CAD build for the part. Positions are in the model's coordinates, mm. Round coordinates to 2 decimals unless told otherwise and drop trailing zeros. Write each loop counter-clockwise with the first axis right and the second up, starting at its lowest first coordinate (ties: lowest second). Pieces come first, ordered by that corner, then holes. Notation, with made-up numbers: (32, 9) - (54, 9) arc R15 cw to (54, 23) - close; hole circle Ø5 at (-7, 4.25). An arc over 180 degrees is marked (long way). Use one line per item in the form item = value. Start each with the question number.
Item 1: Drill centre lines: L1, parallel to Y at x = -12.7, z = -0.75; L2, parallel to Y at x = -10.5, z = -1.4; L3, parallel to X at y = -10, z = 0.25. Where is each one in solid material? Low to high.
Item 2: Band-saw the part on A-A, the plane y = -12.7. List the corners of the cut face in (x, z).
Item 3: Pull direction X, two halves, no side cores. Call faces 1 (the flat face through (-36, 1, -1.588)), 2 (the cylindrical face through (-85.77, 13.71, -0.02)), 3 (the flat face through (0, 1, 0)), 4 (the cylindrical face through (-85.77, -11.69, -0.02)): +X half, -X half, draft (parallel to the pull), parting line (faces both ways), or undercut.
Item 4: Pin check, flat tips, straight feed: pin 1 (1.5 mm diameter, centred on x = -56.5, z = -1, fed in from +Y); pin 2 (5.5 mm diameter, centred on x = -82.55, y = 12.7, fed in from +Z). Stop position of each tip, or through.
Item 5: Band-saw the part on D-D, the plane x = -28.5. List the corners of the cut face in (y, z).
Item 6: Band-saw the part on C-C, the plane x = -82.55. List the corners of the cut face in (y, z), and give its area (3 significant figures).
Item 7: Band-saw the part on B-B, the plane z = -0.1. List the corners of the cut face in (x, y).
from build123d import *

# Parameters (mm, degrees)
BOSS_EXTRUDE3_DEPTH              = 1.5875
F_17_64_0_26563_DIAMETER_HOLE1_D = 6.747002


with BuildPart() as part:
    # Sketch2 → Boss-Extrude3 (new body, symmetric)
    with BuildSketch(Plane.XY):
        Polygon((-95.25, -25.4), (-95.25, 25.4), (0, 76.2), (0, -76.2), align=None)
    extrude(amount=BOSS_EXTRUDE3_DEPTH, both=True)

    # 17/64 (0.26563) Diameter Hole1 (through all)
    with Locations(Plane.XY.offset(1.5875)):
        with Locations((-82.55, 12.7), (-82.55, -12.7), (-12.7, -57.15), (-12.7, 57.15)):
            Hole(F_17_64_0_26563_DIAMETER_HOLE1_D / 2)


solid = part.part
Determined:
q1.L1 = -69.43 to -60.52, -53.78 to 53.78, 60.52 to 69.43
q1.L2 = -70.6 to -59.71, -54.59 to 54.59, 59.71 to 70.6
q1.L3 = -95.25 to -84.57, -80.53 to 0
q2.outline = (-95.25, -1.59) - (-85.92, -1.59) - (-85.92, 1.59) - (-95.25, 1.59) - close; (-79.18, -1.59) - (0, -1.59) - (0, 1.59) - (-79.18, 1.59) - close
q3.face_1 = draft
q3.face_2 = undercut
q3.face_3 = +X half
q3.face_4 = undercut
q4.pin_1 = 46.47
q4.pin_2 = through
q5.outline = (-61, -1.59) - (61, -1.59) - (61, 1.59) - (-61, 1.59) - close
q6.outline = (-32.17, -1.59) - (-16.07, -1.59) - (-16.07, 1.59) - (-32.17, 1.59) - close; (-9.33, -1.59) - (9.33, -1.59) - (9.33, 1.59) - (-9.33, 1.59) - close; (16.07, -1.59) - (32.17, -1.59) - (32.17, 1.59) - (16.07, 1.59) - close
q6.area = 161 mm²
q7.outline = (-95.25, -25.4) - (0, -76.2) - (0, 76.2) - (-95.25, 25.4) - close; hole circle Ø6.75 at (-82.55, -12.7); hole circle Ø6.75 at (-82.55, 12.7); hole circle Ø6.75 at (-12.7, -57.15); hole circle Ø6.75 at (-12.7, 57.15)
